from build123d import *

# Parameters (mm, degrees)
SKETCH_1_R          = 17.5
SKETCH_1_R_2        = 1.25
EXTRUDE_1_DEPTH     = 7
SKETCH_2_R          = 3
CUT_EXTRUDE_1_DEPTH = 3.5


with BuildPart() as part:
    # 草图1 → 凸台-拉伸1 (new body)
    with BuildSketch(Plane.XY):
        Circle(SKETCH_1_R)
        with Locations((0, 7.5)):
            Circle(SKETCH_1_R_2, mode=Mode.SUBTRACT)
        with Locations((7.5, 0)):
            Circle(SKETCH_1_R_2, mode=Mode.SUBTRACT)
        with Locations((0, -7.5)):
            Circle(SKETCH_1_R_2, mode=Mode.SUBTRACT)
        with Locations((-7.5, 0)):
            Circle(SKETCH_1_R_2, mode=Mode.SUBTRACT)
        with Locations((8.838834765, 8.838834765)):
            Circle(SKETCH_1_R_2, mode=Mode.SUBTRACT)
        with Locations((8.838834765, -8.838834765)):
            Circle(SKETCH_1_R_2, mode=Mode.SUBTRACT)
        with Locations((-8.838834765, -8.838834765)):
            Circle(SKETCH_1_R_2, mode=Mode.SUBTRACT)
        with Locations((-8.838834765, 8.838834765)):
            Circle(SKETCH_1_R_2, mode=Mode.SUBTRACT)
    extrude(amount=EXTRUDE_1_DEPTH)

    # 草图2 → 切除-拉伸1 (cut)
    with BuildSketch(Plane.XY.offset(7)):
        with Locations((0, 7.5)):
            Circle(SKETCH_2_R)
        with Locations((7.5, 0)):
            Circle(SKETCH_2_R)
        with Locations((0, -7.5)):
            Circle(SKETCH_2_R)
        with Locations((-7.5, 0)):
            Circle(SKETCH_2_R)
    extrude(amount=-CUT_EXTRUDE_1_DEPTH, mode=Mode.SUBTRACT)


solid = part.part
Build history of the part. All positions in model axes, mm. A direction names the side the tool comes from. Coordinates: 2 decimals unless noted, no trailing zeros. Order: outer loops, then holes, each group sorted by start corner. A loop starts at its lowest first (then second) coordinate and runs counter-clockwise, first axis right, second up. Notation, with made-up numbers: (85, 36.25) - (138, 36.25) arc R20 cw to (138, 60.25) - close; hole circle Ø8 at (-2, 71.25). An arc over 180 degrees is marked (long way). Write each question's results on one line, items separated by ' | '. Start each with the question number.
Item 1: Band-saw the part on A-A on x = 0. Write the cut outline in (y, z), and give its area (4 significant figures).
Item 2: Tool access for faces 4 (the face through (-4.73, -1.15, 5.27)), 5 (the face through (0, 0, 0)): list every direction of +Z, -Z, +X, -X, +Y, -Y with a clear straight run to the whole face (end or side of a thin tool).
Item 3: Flat gauge pins, fed straight in: pin 1 (1 mm diameter, centred on x = -1, z = 1, fed in from -Y); pin 2 (5.5 mm diameter, centred on x = 7.5, y = 0, fed in from +Z); pin 3 (2 mm diameter, centred on x = 8, z = 5.5, fed in from +Y); pin 4 (1.5 mm diameter, centred on x = 8.84, y = -8.84, fed in from -Z). Where does each tip first touch, or does it go through?
Item 4: Band-saw the part on B-B on z = 4.5. State how many separate pieces and enclosed holes the cut face has, and give its area (3 significant figures).
Item 5: Band-saw the part on D-D on x = 7. Write the cut outline in (y, z), and give its area (3 significant figures).
Item 6: Mould opens along X. For faces 1 (the face through (-13.887, -10.648, 3.451)), 2 (the face through (0, -9, 3.5)), 3 (the face through (0, 0, 7)) say: released by +X, released by -X, zero draft, split by the parting line, or undercut.
Item 7: Band-saw the part on C-C on y = 8. Write the cut outline in (x, z).
Item 8: Wall check: probe 1 along X at (y, z) = (-8.5, 0.75); probe 2 along X at (y, z) = (-9, 5.25); probe 3 along Y at (x, z) = (-8, 1.25). Give the ranges that are in metal, low to high. Write a range as [from, to].
Numbers:
1) outline: (-17.5, 0) - (-8.75, 0) - (-8.75, 3.5) - (-10.5, 3.5) - (-10.5, 7) - (-17.5, 7) - close; (-6.25, 0) - (6.25, 0) - (6.25, 3.5) - (4.5, 3.5) - (4.5, 7) - (-4.5, 7) - (-4.5, 3.5) - (-6.25, 3.5) - close; (8.75, 0) - (17.5, 0) - (17.5, 7) - (10.5, 7) - (10.5, 3.5) - (8.75, 3.5) - close | area: 185.5 mm^2
2) face 4: +Z | face 5: -Z, +X, -X, +Y, -Y
3) pin 1: y = -17.49 | pin 2: z = 3.5 | pin 3: y = 16.04 | pin 4: through
4) separate pieces: 1 | enclosed holes: 8 | area: 829 mm^2
5) outline: (-16.04, 0) - (-1.15, 0) - (-1.15, 3.5) - (-2.96, 3.5) - (-2.96, 7) - (-16.04, 7) - close; (1.15, 0) - (16.04, 0) - (16.04, 7) - (2.96, 7) - (2.96, 3.5) - (1.15, 3.5) - close | area: 196 mm^2
6) face 1: split by the parting line | face 2: undercut | face 3: zero draft
7) outline: (-15.56, 0) - (-9.77, 0) - (-9.77, 7) - (-15.56, 7) - close; (-7.91, 0) - (-1.15, 0) - (-1.15, 3.5) - (-2.96, 3.5) - (-2.96, 7) - (-7.91, 7) - close; (1.15, 0) - (7.91, 0) - (7.91, 7) - (2.96, 7) - (2.96, 3.5) - (1.15, 3.5) - close; (9.77, 0) - (15.56, 0) - (15.56, 7) - (9.77, 7) - close
8) probe 1: [-15.3, -10.04], [-7.64, -0.75], [0.75, 7.64], [10.04, 15.3] | probe 2: [-15.01, -10.08], [-7.6, -2.6], [2.6, 7.6], [10.08, 15.01] | probe 3: [-15.56, -9.77], [-7.91, -1.15], [1.15, 7.91], [9.77, 15.56]
